Part model, mm, in its own coordinate system. A direction names the side the tool comes from. Give positions to 0.01 mm unless a question says otherwise; leave off trailing zeros. Write each loop counter-clockwise with the first axis right and the second up, starting at its lowest first coordinate (ties: lowest second). Pieces come first, ordered by that corner, then holes.
Autodesk Inventor part; units mm, degrees
ref_plane "YZ Plane" through (0, 0, 0) normal (1, 0, 0) x (0, 1, 0)
ref_plane "XZ Plane" through (0, 0, 0) normal (0, 1, 0) x (-1, 0, 0)
ref_plane "XY Plane" through (0, 0, 0) normal (0, 0, 1) x (1, 0, 0)
sketch "スケッチ1" plane through (0, 0, 0) normal (0, 1, 0) x (-1, 0, 0)
  circle A0 centre (0, 0) radius 3
  dimension "d0" = 6
extrude "押し出し1" add sketch "スケッチ1" along normal blind 115
ref_plane "作業平面1" through (0, 57.5, 0) normal (0, 1, 0) x (1, 0, 0)
sketch "スケッチ2" plane through (0, 57.5, 0) normal (0, 1, 0) x (1, 0, 0)
  circle A0 centre (0, 0) radius 5
  dimension "d3" = 10
extrude "押し出し2" add sketch "スケッチ2" along normal blind 13.9 and the other way blind 13.9
sketch "スケッチ4" plane through (0, 43.6, 0) normal (0, -1, 0) x (1, 0, 0)
  circle A0 centre (0, 0) radius 4
  dimension "d9" = 8
extrude "押し出し3" add sketch "スケッチ4" along normal blind 32
sketch "スケッチ5" plane through (0, 71.4, 0) normal (0, 1, 0) x (1, 0, 0)
  circle A0 centre (0, 0) radius 4
  dimension "d12" = 8
extrude "押し出し4" add sketch "スケッチ5" along normal blind 19
properties part number "shoulder1_shaft copy"
1) Saw through at A-A, the plane x = 0. Write the cut outline in (y, z).
Answers follow:
outline: (0, -3) - (11.6, -3) - (11.6, -4) - (43.6, -4) - (43.6, -5) - (71.4, -5) - (71.4, -4) - (90.4, -4) - (90.4, -3) - (115, -3) - (115, 3) - (90.4, 3) - (90.4, 4) - (71.4, 4) - (71.4, 5) - (43.6, 5) - (43.6, 4) - (11.6, 4) - (11.6, 3) - (0, 3) - close
2) 3-axis set-ups, long thin cutter, end or side, ignore diameter. For faces 1 (the face through (0, 0, 0)), 2 (the face through (1, 11.6, 3)), 3 (the face through (1, 90.4, -3)): which of +Z, -Z, +X, -X, +Y, -Y reach the whole face in a straight line?
Answers follow:
face 1: +Z, -Z, +X, -X, -Y
face 2: -Y
face 3: +Y
3) Wall check: L1, parallel to Y at x = 2.5, z = 2.75; L2, parallel to Z at x = 0.25, y = 96; L3, parallel to X at y = 65, z = 3. Give the ranges that are in metal, low to high.
Answers follow:
L1: y = 11.6 to 90.4
L2: z = -2.99 to 2.99
L3: x = -4 to 4
4) Saw through at C-C, the plane y = 93. Write the cut outline in (x, z), then the cut area to 3 significant figures.
Answers follow:
outline: circle Ø6 at (0, 0)
area: 28.3 mm2
5) Pin check, flat tips, straight feed: pin 1 Ø4 at (y, z) = (26, -1.5) entering from -X; pin 2 Ø1.5 at (x, z) = (4, 1.5) entering from -Y; pin 3 Ø5 at (x, y) = (-3.5, 55) entering from +Z. Stop position of each tip, or through.
Answers follow:
pin 1: stops at x = -4
pin 2: stops at y = 11.6
pin 3: stops at z = 4.9
6) Saw through at B-B, the plane z = 0. Write the cut outline in (x, y), then the cut area to 3 significant figures.
Answers follow:
outline: (-5, 43.6) - (-4, 43.6) - (-4, 11.6) - (-3, 11.6) - (-3, 0) - (3, 0) - (3, 11.6) - (4, 11.6) - (4, 43.6) - (5, 43.6) - (5, 71.4) - (4, 71.4) - (4, 90.4) - (3, 90.4) - (3, 115) - (-3, 115) - (-3, 90.4) - (-4, 90.4) - (-4, 71.4) - (-5, 71.4) - close
area: 903 mm2
